```python
from build123d import *

# Parameters (mm, degrees)
F0_W      = 355.6
F0_H      = 215.9
F1_DEPTH  = 6.35
F2_R      = 1.778
F3_DEPTH  = 6.351
F4_R      = 0.79375
F5_DEPTH  = 6.351
F6_R      = 1.778
F7_DEPTH  = 6.351
F8_R      = 1.2192
F9_DEPTH  = 6.351
F10_W     = 342.9
F10_H     = 203.2
F10_W_2   = 165.1127
F10_H_2   = 114.8461
F10_W_3   = 145.7325
F10_H_3   = 95.5675
F10_W_4   = 145.1737
F10_H_4   = 95.0087
F11_DEPTH = 0.2794


with BuildPart() as f1:
    # F0 (on Top) → F1 (new body)
    with BuildSketch(Plane.XY):
        with Locations((177.8, 107.95)):
            Rectangle(F0_W, F0_H)
    extrude(amount=F1_DEPTH)

    # F2 (on face) → F3 (cut, through all)
    with BuildSketch(Plane.XY.offset(6.35)):
        with Locations((3.175, 107.95)):
            Circle(F2_R)
        with Locations((3.108338, 25.400027)):
            Circle(F2_R)
        with Locations((3.108338, 190.499973)):
            Circle(F2_R)
        with Locations((177.8, 3.175)):
            Circle(F2_R)
        with Locations((330.2, 3.175)):
            Circle(F2_R)
        with Locations((330.2, 212.725)):
            Circle(F2_R)
        with Locations((25.4, 3.175)):
            Circle(F2_R)
        with Locations((177.8, 212.725)):
            Circle(F2_R)
        with Locations((25.4, 212.725)):
            Circle(F2_R)
        with Locations((352.491662, 190.499973)):
            Circle(F2_R)
        with Locations((352.425, 107.95)):
            Circle(F2_R)
        with Locations((352.491662, 25.400027)):
            Circle(F2_R)
    extrude(amount=-F3_DEPTH, mode=Mode.SUBTRACT)

    # F4 (on face) → F5 (cut, through all)
    with BuildSketch(Plane.XY.offset(6.35)):
        with Locations((127, 107.95)):
            Circle(F4_R)
        with Locations((61.9125, 78.35265)):
            Circle(F4_R)
        with Locations((192.0875, 78.35265)):
            Circle(F4_R)
        with Locations((61.9125, 137.54735)):
            Circle(F4_R)
        with Locations((192.0875, 137.54735)):
            Circle(F4_R)
    extrude(amount=-F5_DEPTH, mode=Mode.SUBTRACT)

    # F6 (on face) → F7 (cut, through all)
    with BuildSketch(Plane.XY.offset(6.35)):
        with Locations((204.62875, 155.7274)):
            Circle(F6_R)
        with Locations((204.62875, 60.1726)):
            Circle(F6_R)
        with Locations((194.4878, 55.245)):
            Circle(F6_R)
        with Locations((61.1378, 55.245)):
            Circle(F6_R)
    extrude(amount=-F7_DEPTH, mode=Mode.SUBTRACT)

    # F8 (on face) → F9 (cut, through all)
    with BuildSketch(Plane.XY.offset(6.35)):
        with Locations((82.55, 160.3375)):
            Circle(F8_R)
        with Locations((127, 160.3375)):
            Circle(F8_R)
        with Locations((171.45, 160.3375)):
            Circle(F8_R)
        with Locations((82.55, 55.5625)):
            Circle(F8_R)
        with Locations((127, 55.5625)):
            Circle(F8_R)
        with Locations((171.45, 55.5625)):
            Circle(F8_R)
        with Locations((204.62875, 139.7)):
            Circle(F8_R)
        with Locations((204.62875, 76.2)):
            Circle(F8_R)
        with Locations((204.62875, 107.95)):
            Circle(F8_R)
        with Locations((49.37125, 139.7)):
            Circle(F8_R)
        with Locations((49.37125, 107.95)):
            Circle(F8_R)
        with Locations((49.37125, 76.2)):
            Circle(F8_R)
    extrude(amount=-F9_DEPTH, mode=Mode.SUBTRACT)

    # F10 (on face) → F11 (cut)
    with BuildSketch(Plane.XY.offset(6.35)):
        with Locations((177.8, 107.95)):
            Rectangle(F10_W, F10_H)
        with Locations((127, 107.79125)):
            Rectangle(F10_W_2, F10_H_2, mode=Mode.SUBTRACT)
        with Locations((127, 107.79125)):
            Rectangle(F10_W_3, F10_H_3)
        with Locations((127, 107.79125)):
            Rectangle(F10_W_4, F10_H_4, mode=Mode.SUBTRACT)
    extrude(amount=-F11_DEPTH, mode=Mode.SUBTRACT)


solid = f1.part
```
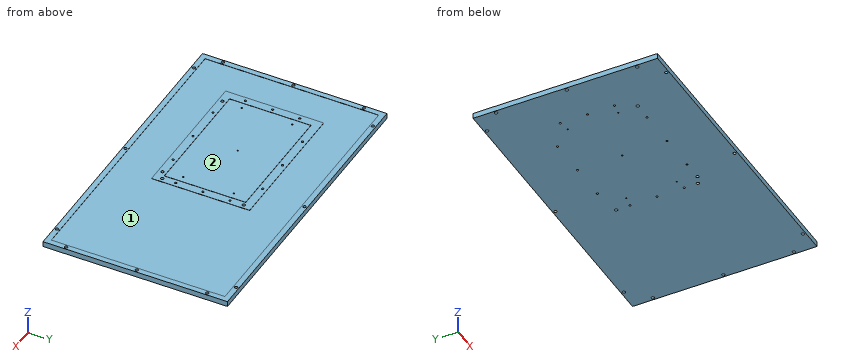
The listing builds one solid part. Answer for the finished solid, in the listing's coordinates (mm). Face numbers are marked on the shaded views. Round coordinates to 2 decimals unless told otherwise and drop trailing zeros. Write each loop counter-clockwise with the first axis right and the second up, starting at its lowest first coordinate (ties: lowest second). Pieces come first, ordered by that corner, then holes. Notation, with made-up numbers: (-20, 42.25) -> (9, 42.25) arc R37 ccw to (9, 79.25) -> close; hole circle Ø7 at (86.5, -30.5). An arc over 180 degrees is marked (long way). Use CSV: the item, a comma, the result in double quotes. Start each with the question number.
(1) Consider L1, parallel to X at y = 76.2, z = 2.25; L2, parallel to Y at x = 249, z = 6.25; L3, parallel to Y at x = 82.55, z = 3. Determine where each line is inside the solid, lowest interval first. Write a range as from..to.
(2) The mould has two halves that part along X. Classify the marked faces 1 and 2: released by +X, released by -X, zero draft, split by the parting line, or undercut.
(3) Section B-B on x = 282.5 is taken. Give the vertices of the cut face in (y, z), then the cut area to 3 significant figures.
(4) Section A-A on y = 93.5 is taken. Give the vertices of the cut face in (x, z).
(5) This flat-tipped pin is pushed along its axis until it touches: pin 1 (5 mm diameter, centred on x = 221.5, y = 139.5, fed in from +Z). Where does it stop, or does it pass through?
(6) Section C-C on y = 41.5 is taken. Give the vertices of the cut face in (x, z), then the cut area to 3 significant figures.
A:
1,L1,"x = 0..48.15, 50.59..203.41, 205.85..355.6"
1,L2,"y = 0..6.35, 209.55..215.9"
1,L3,"y = 0..54.34, 56.78..159.12, 161.56..215.9"
2,face 1,"undercut"
2,face 2,"zero draft"
3,outline,"(0, 0) -> (215.9, 0) -> (215.9, 6.35) -> (209.55, 6.35) -> (209.55, 6.07) -> (6.35, 6.07) -> (6.35, 6.35) -> (0, 6.35) -> close"
3,area,"1,310 mm²"
4,outline,"(0, 0) -> (355.6, 0) -> (355.6, 6.35) -> (349.25, 6.35) -> (349.25, 6.07) -> (209.56, 6.07) -> (209.56, 6.35) -> (199.87, 6.35) -> (199.87, 6.07) -> (199.59, 6.07) -> (199.59, 6.35) -> (54.41, 6.35) -> (54.41, 6.07) -> (54.13, 6.07) -> (54.13, 6.35) -> (44.44, 6.35) -> (44.44, 6.07) -> (6.35, 6.07) -> (6.35, 6.35) -> (0, 6.35) -> close"
5,pin 1,"stops at z = 6.07"
6,outline,"(0, 0) -> (355.6, 0) -> (355.6, 6.35) -> (349.25, 6.35) -> (349.25, 6.07) -> (6.35, 6.07) -> (6.35, 6.35) -> (0, 6.35) -> close"
6,area,"2,160 mm²"
